For this review, take the finished solid that the model builds, in its own axes (mm). Coordinates: 2 decimals unless noted, no trailing zeros. Write each loop counter-clockwise with the first axis right and the second up, starting at its lowest first coordinate (ties: lowest second). Pieces come first, ordered by that corner, then holes.
Autodesk Inventor part; units mm, degrees
ref_plane "YZ Plane" through (0, 0, 0) normal (1, 0, 0) x (0, 1, 0)
ref_plane "XZ Plane" through (0, 0, 0) normal (0, 1, 0) x (-1, 0, 0)
ref_plane "XY Plane" through (0, 0, 0) normal (0, 0, 1) x (1, 0, 0)
sketch "Sketch1" plane through (0, 0, 0) normal (0, 0, 1) x (1, 0, 0)
  line L0 (0, 0) -> (63.5, 0)
  line L1 (0, 0) -> (0, 63.5)
  line L2 (0, 63.5) -> (63.5, 0)
  dimension "d0" = 63.5
  dimension "d1" = 63.5
extrude "Extrusion1" add sketch "Sketch1" along normal mid plane 3.175
fillet "Fillet1" radius 3.175 3 edges at (0, 63.5, 0) (63.5, 0, 0) (0, 0, 0)
sketch "Sketch2" plane through (0, 0, 1.5875) normal (0, 0, 1) x (1, 0, 0)
  arc A0 (0, 3.175) -> (3.175, 0) centre (3.175, 3.175) ccw construction
  line L0 (0, 3.175) -> (0, 55.8349) construction
  arc A1 (5.4201, 58.0799) -> (0, 55.8349) centre (3.175, 55.8349) ccw construction
  line L1 (5.4201, 58.0799) -> (58.0799, 5.4201) construction
  arc A2 (55.8349, 0) -> (58.0799, 5.4201) centre (55.8349, 3.175) ccw construction
  line L2 (55.8349, 0) -> (3.175, 0) construction
  point P0 (0, 0)
  point P1 (12.7, 12.7)
  dimension "d5" = 12.7
  dimension "d6" = 12.7
hole "Hole1" at (12.7, 12.7, 1.5875) direction (0, 0, -1) diameter 5.1054 end through all
pattern_linear "Rectangular Pattern1" count 2 spacing 25.4 along (1, 0, 0) of "Hole1"
pattern_linear "Rectangular Pattern2" count 2 spacing 25.4 along (0, 1, 0) of "Hole1"
equation "\"d1\" = d0"
properties part number "EL2-C-002" material "Aluminum 6061"
1) The part is to be moulded in two halves that separate along Y. For faces 1 (the face through (58.748, 1.912, 0.022)), 2 (the face through (1.912, 58.748, -0.022)), 3 (the face through (35.57, 13.03, -0.02)), say which applies: pulls with the +Y half, pulls with the -Y half, needs draft (parallel to the pull), parting line crosses it, or undercut.
2) For L1, parallel to X at y = 12.7, z = 0.4; L2, parallel to Y at x = 12.5, z = 1.1, list the stretches that pass through material, from the lowest coordinate up.
3) Consider section A-A (y = 12.7). Give the boundary of the cut face in (x, z).
4) Consider section C-C (x = 38.1). Give the boundary of the cut face in (y, z), then the cut area to 3 significant figures.
5) Consider section B-B (z = 0.3). Give the boundary of the cut face in (x, y) (3 decimals).
Results:
1. face 1: parting line crosses it
1. face 2: pulls with the +Y half
1. face 3: undercut
2. L1: x = 0 to 10.15, 15.25 to 35.55, 40.65 to 50.8
2. L2: y = 0 to 10.16, 15.24 to 35.56, 40.64 to 51
3. outline: (0, -1.59) - (10.15, -1.59) - (10.15, 1.59) - (0, 1.59) - close; (15.25, -1.59) - (35.55, -1.59) - (35.55, 1.59) - (15.25, 1.59) - close; (40.65, -1.59) - (50.8, -1.59) - (50.8, 1.59) - (40.65, 1.59) - close
4. outline: (0, -1.59) - (10.15, -1.59) - (10.15, 1.59) - (0, 1.59) - close; (15.25, -1.59) - (25.4, -1.59) - (25.4, 1.59) - (15.25, 1.59) - close
4. area: 64.4 mm2
5. outline: (0, 3.175) arc R3.175 ccw to (3.175, 0) - (55.835, 0) arc R3.175 ccw to (58.08, 5.42) - (5.42, 58.08) arc R3.175 ccw to (0, 55.835) - close; hole circle Ø5.105 at (12.7, 12.7); hole circle Ø5.105 at (12.7, 38.1); hole circle Ø5.105 at (38.1, 12.7)
